CAD build for the part. Positions are in the model's coordinates, mm. A direction names the side the tool comes from. Round coordinates to 2 decimals unless told otherwise and drop trailing zeros. Loops run counter-clockwise (first coordinate to the right, second up) from the corner with the lowest first, then second, coordinate; pieces in that order, holes last. Notation, with made-up numbers: (56.5, -28) - (80.5, -28) arc R12 ccw to (80.5, -5) - close; hole circle Ø9 at (39, 1.25). An arc over 180 degrees is marked (long way). Use one line per item in the form item = value.
from build123d import *

# Parameters (mm, degrees)
SKETCH_2_R      = 0.75
EXTRUDE_1_DEPTH = 1


with BuildPart() as part:
    # Эскиз2 → Бобышка-Вытянуть1 (new body)
    with BuildSketch(Plane.XY):
        with BuildLine():
            Line((1e-09, 4.75), (0, 6.55))
            ThreePointArc((0, 6.55), (-5.174962188, 3.628926318), (-5.348211601, -2.311013895))
            ThreePointArc((-5.348211601, -2.311013895), (-5.179687707, -3.123034993), (-5.468378103, -3.900490086))
            ThreePointArc((-5.468378103, -3.900490086), (-4.719418002, -6.425234093), (-2.496065251, -5.013860266))
            Line((-2.496065251, -5.013860266), (-2.468043041, -4.670176577))
            ThreePointArc((-2.468043041, -4.670176577), (-2.552204681, -4.179903536), (-2.862172849, -3.790839825))
            ThreePointArc((-2.862172849, -3.790839825), (-4.503831101, 1.50930627), (1e-09, 4.75))
        make_face()
        with Locations((-4.140632757, -4.880077906)):
            Circle(SKETCH_2_R, mode=Mode.SUBTRACT)
    extrude(amount=EXTRUDE_1_DEPTH)

    # Зеркальное отражение1: part across plane


with BuildPart() as part_1:
    add(part.part)
    add(part.part.mirror(Plane(origin=(1e-09, 4.75, 1), x_dir=(0, 0, 1), z_dir=(-1, 0, 0))))


solid = part_1.part
1) Drill centre lines: probe 1 along Y at (x, z) = (4, 0.15); probe 2 along X at (y, z) = (-5.25, 0.7); probe 3 along Y at (x, z) = (-4.25, 0.5). Where is each one in solid material? Low to high.
Report:
probe_1 = -6.52 to -5.62, -4.14 to -2.56, 2.56 to 5.04
probe_2 = -5.75 to -4.79, -3.49 to -2.53, 2.53 to 3.49, 4.79 to 5.75
probe_3 = -6.53 to -5.62, -4.14 to -2.12, 2.12 to 4.8
2) Two-plate mould, pull along X, no slides. Class faces 1 (the flat face through (0, 5, 1)), 2 (the cylindrical face through (-4.89, -4.85, 0.49)), 3 (the cylindrical face through (4.76, -6.41, 0.49)), 4 (the cylindrical face through (-5.18, -3.11, 0.49)): +X half, -X half, draft (parallel to the pull), parting line (faces both ways), or undercut.
Report:
face_1 = draft
face_2 = undercut
face_3 = undercut
face_4 = -X half
3) Slice it at B-B (z = 0.75). Write the cut outline in (x, y), plus the area to 3 significant figures.
Report:
outline = (-5.47, -3.9) arc R1.65 ccw (long way) to (-2.5, -5.01) - (-2.47, -4.67) arc R1 ccw to (-2.86, -3.79) arc R4.75 cw (long way) to (2.86, -3.79) arc R1 ccw to (2.47, -4.67) - (2.5, -5.01) arc R1.65 ccw (long way) to (5.47, -3.9) arc R1.5 cw to (5.35, -2.31) arc R6.04 ccw (long way) to (-5.35, -2.31) arc R1.5 cw to start; hole circle Ø1.5 at (-4.14, -4.88); hole circle Ø1.5 at (4.14, -4.88)
area = 50.3 mm^2
4) Slice it at C-C (y = -1.25). Write the cut outline in (x, z).
Report:
outline = (-5.78, 0) - (-4.58, 0) - (-4.58, 1) - (-5.78, 1) - close; (4.58, 0) - (5.78, 0) - (5.78, 1) - (4.58, 1) - close
5) Tool access for faces 5 (the cylindrical face through (2.549, -4.186, 0.493)), 6 (the flat face through (0, 5, 0)): list every direction of +Z, -Z, +X, -X, +Y, -Y with a clear straight run to the whole face (end or side of a thin tool).
Report:
face_5 = +Z, -Z
face_6 = -Z, +X, -X, +Y, -Y
6) Slice it at D-D (x = 2). Write the cut outline in (y, z).
Report:
outline = (4.31, 0) - (6.21, 0) - (6.21, 1) - (4.31, 1) - close
7) Flat gauge pin, fed straight in: pin 1 (0.9 mm diameter, centred on x = -4.14, y = -4.88, fed in from +Z). Where does the tip first touch, or does it go through?
Report:
pin_1 = through
8) Slice it at A-A (y = -3.25). Write the cut outline in (x, z), plus the area to 3 significant figures.
Report:
outline = (-5.19, 0) - (-3.46, 0) - (-3.46, 1) - (-5.19, 1) - close; (3.46, 0) - (5.19, 0) - (5.19, 1) - (3.46, 1) - close
area = 3.46 mm^2
